```python
from build123d import *

# Parameters (mm, degrees)
F0_R     = 10
F0_W     = 0.8
F0_H     = 2
F0_R_2   = 1.5
F0_R_3   = 0.25
F1_DEPTH = 3
F2_DEPTH = 1.5


with BuildPart() as f1:
    # F0 (on Top) → F1 (new body)
    with BuildSketch(Plane.XY):
        Circle(F0_R)
        with Locations((-9, 0)):
            Rectangle(F0_W, F0_H, mode=Mode.SUBTRACT)
        with Locations((-6.5, 0)):
            Circle(F0_R_2, mode=Mode.SUBTRACT)
        with Locations((-1.75, 0)):
            Circle(F0_R_3, mode=Mode.SUBTRACT)
        with Locations((1.5, 0)):
            Circle(F0_R_3, mode=Mode.SUBTRACT)
        with Locations((9, 0)):
            Rectangle(F0_W, F0_H, mode=Mode.SUBTRACT)
    extrude(amount=F1_DEPTH)

    # F0 (on Top) → F2 (join)
    with BuildSketch(Plane.XY):
        with Locations((-9, 0)):
            Rectangle(F0_W, F0_H)
        with Locations((9, 0)):
            Rectangle(F0_W, F0_H)
    extrude(amount=F2_DEPTH)


solid = f1.part
```
Build history of the part. All positions in model axes, mm. A direction names the side the tool comes from. Give positions to 0.01 mm unless a question says otherwise; leave off trailing zeros. Loops run counter-clockwise (first coordinate to the right, second up) from the corner with the lowest first, then second, coordinate; pieces in that order, holes last.
1) Drop flat-ended pins along their axis: P1, Ø0.6, axis at x = -9, z = 2, coming from the +Y side; P2, Ø1, axis at x = 6.5, z = 1, coming from the -Y side; P3, Ø0.6, axis at x = -9, z = 2.5, coming from the -Y side. Give the stop position or say it passes through.
Values follow:
P1: stops at y = 4.93
P2: stops at y = -8
P3: stops at y = -4.93
2) Two-plate mould, pull along Y, no slides. Class faces 3 (the face through (9.4, 0, 2)), 4 (the face through (0, 0, 3)), 5 (the face through (-2.17, -9.76, 1.48)): released by +Y, released by -Y, zero draft, split by the parting line, or undercut.
Values follow:
face 3: undercut
face 4: zero draft
face 5: split by the parting line
3) Band-saw the part on B-B on x = -1.75. List the corners of the cut face in (y, z), then the cut area to 3 significant figures.
Values follow:
outline: (-9.85, 0) - (-0.25, 0) - (-0.25, 3) - (-9.85, 3) - close; (0.25, 0) - (9.85, 0) - (9.85, 3) - (0.25, 3) - close
area: 57.6 mm2
4) Band-saw the part on A-A on y = 0. List the corners of the cut face in (x, z).
Values follow:
outline: (-10, 0) - (-8, 0) - (-8, 3) - (-8.6, 3) - (-8.6, 1.5) - (-9.4, 1.5) - (-9.4, 3) - (-10, 3) - close; (-5, 0) - (-2, 0) - (-2, 3) - (-5, 3) - close; (-1.5, 0) - (1.25, 0) - (1.25, 3) - (-1.5, 3) - close; (1.75, 0) - (10, 0) - (10, 3) - (9.4, 3) - (9.4, 1.5) - (8.6, 1.5) - (8.6, 3) - (1.75, 3) - close
5) Band-saw the part on D-D on z = 1.2. List the corners of the cut face in (x, y), then the cut area to 3 significant figures.
Values follow:
outline: circle Ø20 at (0, 0); hole circle Ø3 at (-6.5, 0); hole circle Ø0.5 at (-1.75, 0); hole circle Ø0.5 at (1.5, 0)
area: 307 mm2
6) Band-saw the part on C-C on z = 2.6. List the corners of the cut face in (x, y), then the cut area to 3 significant figures.
Values follow:
outline: circle Ø20 at (0, 0); hole (-9.4, -1) - (-8.6, -1) - (-8.6, 1) - (-9.4, 1) - close; hole circle Ø3 at (-6.5, 0); hole circle Ø0.5 at (-1.75, 0); hole circle Ø0.5 at (1.5, 0); hole (8.6, -1) - (9.4, -1) - (9.4, 1) - (8.6, 1) - close
area: 303 mm2
7) Probe line 1 along Y through (x, z) = (-6.5, 2.15); line 2 along Y through (x, z) = (1.5, 1.8); line 3 along Y through (x, z) = (-0.5, 1.35). List the from-to ranges inside material, lowest first.
Values follow:
line 1: y = -7.6 to -1.5, 1.5 to 7.6
line 2: y = -9.89 to -0.25, 0.25 to 9.89
line 3: y = -9.99 to 9.99
8) 3-axis set-ups, long thin cutter, end or side, ignore diameter. For faces 1 (the face through (0, 0, 0)), 2 (the face through (9, -1, 2)): which of +Z, -Z, +X, -X, +Y, -Y reach the whole face in a straight line?
Values follow:
face 1: -Z, +X, -X, +Y, -Y
face 2: +Z
